Geometry: see drawing. Coordinates: mm, zero at the bounding-box minimum. Coordinates: 2 decimals unless noted, no trailing zeros. Write each loop counter-clockwise with the first axis right and the second up, starting at its lowest first coordinate (ties: lowest second). Pieces come first, ordered by that corner, then holes.
1) Section query A-A (z = 63.5). Output: boundary loops of the cut face in (x, y), then the cut area to 3 significant figures.
2) Pin query (flat end, axial travel): pin 1 Ø12 at (x, z) = (205, 112.5) entering from -Y. Return the tip coordinate at first contact, or that it passes through.
3) Line query: L1, parallel to Y at x = 293, z = 84. Output: solid intervals per line, ascending.
4) Section query C-C (z = 116.5). Output: boundary loops of the cut face in (x, y), then the cut area to 3 significant figures.
5) Section query B-B (x = 337.5). Output: boundary loops of the cut face in (y, z), then the cut area to 3 significant figures.
6) Section query D-D (x = 271). Output: boundary loops of the cut face in (y, z), then the cut area to 3 significant figures.
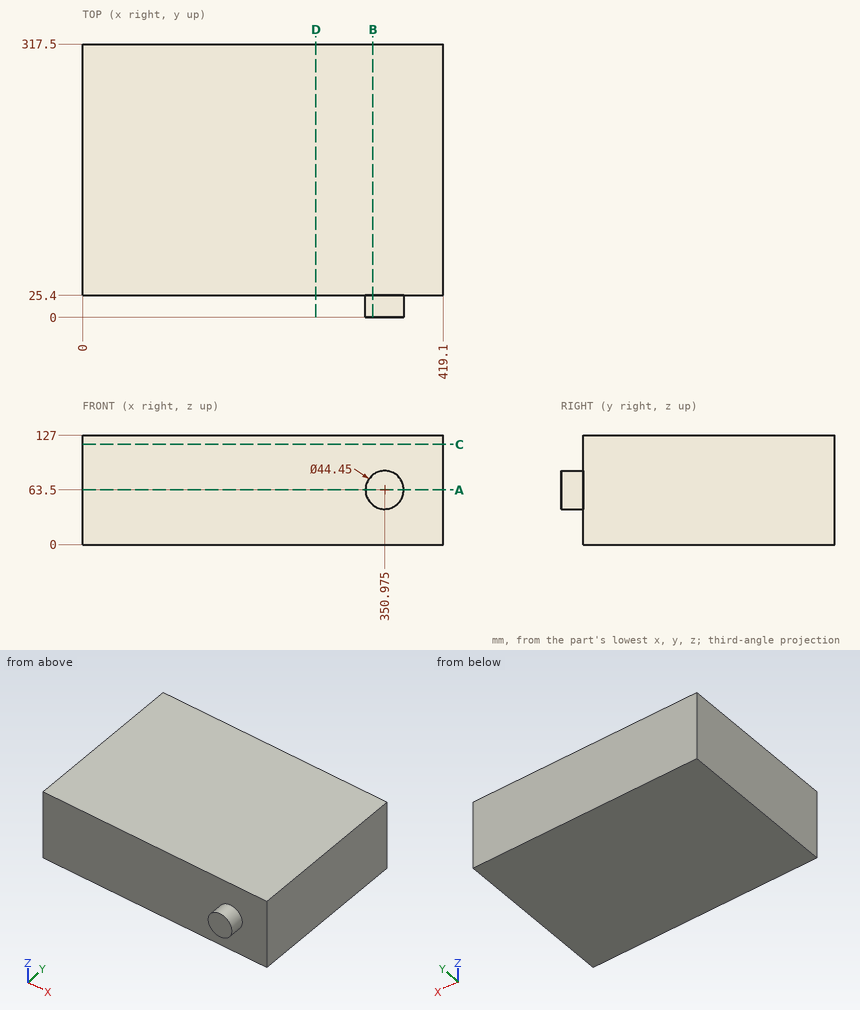
Answer:
1. outline: (0, 25.4) - (328.75, 25.4) - (328.75, 0) - (373.2, 0) - (373.2, 25.4) - (419.1, 25.4) - (419.1, 317.5) - (0, 317.5) - close
1. area: 124,000 mm2
2. pin 1: stops at y = 25.4
3. L1: y = 25.4 to 317.5
4. outline: (0, 25.4) - (419.1, 25.4) - (419.1, 317.5) - (0, 317.5) - close
4. area: 122,000 mm2
5. outline: (0, 45.83) - (25.4, 45.83) - (25.4, 0) - (317.5, 0) - (317.5, 127) - (25.4, 127) - (25.4, 81.17) - (0, 81.17) - close
5. area: 38,000 mm2
6. outline: (25.4, 0) - (317.5, 0) - (317.5, 127) - (25.4, 127) - close
6. area: 37,100 mm2
